Read the model definition and answer for the solid it produces. Units are mm, in the model's axes. Coordinates: 2 decimals unless noted, no trailing zeros. Order: outer loops, then holes, each group sorted by start corner. A loop starts at its lowest first (then second) coordinate and runs counter-clockwise, first axis right, second up. Notation, with made-up numbers: (43.5, 68.5) -> (101.5, 68.5) arc R13 ccw to (101.5, 74.5) -> close; hole circle Ø4 at (74, -31.5). An arc over 180 degrees is marked (long way). Answer as a JSON object with one key per item and string values. Group by question number.
1) Determine the mould class of faces 1 (the cylindrical face through (39.1, 0.86, 0.99)), 2 (the cylindrical face through (0.86, 0.9, 0.99)), 3 (the cylindrical face through (27.776, 30.775, 1.479)), 4 (the cylindrical face through (19.762, 39.715, 2.699)) for opening direction X: released by +X, released by -X, zero draft, split by the parting line, or undercut.
2) Section D-D on y = 36 is taken. Determine the outline of the cut face in (x, z).
3) Section B-B on x = 29 is taken. Determine the outline of the cut face in (y, z), and give its area (3 significant figures).
4) Consider L1, parallel to Y at x = 15.5, z = 2.3; L2, parallel to Y at x = 26, z = 0.85; L3, parallel to X at y = 24.5, z = 1.65. Determine where each line is inside the solid, lowest interval first.
5) Section C-C on x = 36 is taken. Determine the outline of the cut face in (y, z).
6) Section A-A on y = 30 is taken. Determine the outline of the cut face in (x, z), and give its area (3 significant figures).
7) Given pin 1 (19 mm diameter, centred on x = 22, y = 23.5, fed in from +Z); pin 2 (4.5 mm diameter, centred on x = 4, y = 36, fed in from +Z); pin 3 (4 mm diameter, centred on x = 24.5, y = 25, fed in from +Z), each flat-ended and moving along its own axis, determine where each tip first touches the part or whether it passes through.
from build123d import *

# Parameters (mm, degrees)
F0_R     = 1.75
F1_DEPTH = 3
F2_R     = 1


with BuildPart() as f1:
    # F0 (on Top) → F1 (new body)
    with BuildSketch(Plane.XY):
        with BuildLine():
            ThreePointArc((0, 3), (0.8786796564, 0.8786796564), (3, 0))
            Line((3, 0), (37, 0))
            ThreePointArc((37, 0), (39.1213203436, 0.8786796564), (40, 3))
            Line((40, 3), (40, 37))
            ThreePointArc((40, 37), (39.1213203436, 39.1213203436), (37, 40))
            Line((37, 40), (3, 40))
            ThreePointArc((3, 40), (0.8786796564, 39.1213203436), (0, 37))
            Line((0, 37), (0, 3))
        make_face()
        with Locations((4, 4)):
            Circle(F0_R, mode=Mode.SUBTRACT)
        with BuildLine():
            ThreePointArc((25.7168143959, 2.4054544485), (16.6516253204, 1.8055396616), (8.3939355728, 5.5934296756))
            ThreePointArc((8.3939355728, 5.5934296756), (20.1917154021, 6.7967188392), (27.1456707418, 16.4028636876))
            ThreePointArc((27.1456707418, 16.4028636876), (27.9768447331, 19.3917664063), (27.6084521304, 22.472135955))
            ThreePointArc((27.6084521304, 22.472135955), (31.4294663136, 11.9894373312), (25.7168143959, 2.4054544485))
        make_face(mode=Mode.SUBTRACT)
        with BuildLine():
            ThreePointArc((5.0331856041, 9.1259728326), (1.6613352552, 17.56209611), (2.7120662697, 26.5861481412))
            ThreePointArc((2.7120662697, 26.5861481412), (7.5021767329, 15.7376295574), (18.7870537655, 12.0924870261))
            ThreePointArc((18.7870537655, 12.0924870261), (21.8865160613, 12.2256153201), (24.7022820183, 13.527864045))
            ThreePointArc((24.7022820183, 13.527864045), (15.9134015021, 6.6545315855), (5.0331856041, 9.1259728326))
        make_face(mode=Mode.SUBTRACT)
        with Locations((36, 4)):
            Circle(F0_R, mode=Mode.SUBTRACT)
        with BuildLine():
            ThreePointArc((20, 28), (31.1503971529, 28.3946684161), (38.5, 20))
            ThreePointArc((38.5, 20), (36.2692553858, 11.1931089939), (30.1149914386, 4.5101017371))
            ThreePointArc((30.1149914386, 4.5101017371), (32.6163099018, 16.1022939223), (25.6292136254, 25.6843604706))
            ThreePointArc((25.6292136254, 25.6843604706), (23.0434451067, 27.3984756459), (20, 28))
        make_face(mode=Mode.SUBTRACT)
        with BuildLine():
            ThreePointArc((5.0331856041, 30.8740271674), (12.014456559, 36.687752873), (20.9215337867, 38.4770337306))
            ThreePointArc((20.9215337867, 38.4770337306), (12.0842050334, 30.5689913546), (12.1046872588, 18.7100245281))
            ThreePointArc((12.1046872588, 18.7100245281), (13.1890863131, 15.8033996199), (15.2977179817, 13.527864045))
            ThreePointArc((15.2977179817, 13.527864045), (6.0448769164, 19.7626095929), (5.0331856041, 30.8740271674))
        make_face(mode=Mode.SUBTRACT)
        with Locations((4, 36)):
            Circle(F0_R, mode=Mode.SUBTRACT)
        with BuildLine():
            ThreePointArc((25.7168143959, 37.5945455515), (33.4033274796, 32.7515023614), (37.8574729322, 24.8332867156))
            ThreePointArc((37.8574729322, 24.8332867156), (27.6055929298, 30.7943663266), (16.3333746086, 27.1102642876))
            ThreePointArc((16.3333746086, 27.1102642876), (13.9041077858, 25.1807430078), (12.3915478696, 22.472135955))
            ThreePointArc((12.3915478696, 22.472135955), (15.461858115, 33.1987530743), (25.7168143959, 37.5945455515))
        make_face(mode=Mode.SUBTRACT)
        with Locations((36, 36)):
            Circle(F0_R, mode=Mode.SUBTRACT)
    extrude(amount=F1_DEPTH)

    # F2
    f2_edges = [f1.edges().sort_by_distance(p)[0] for p in [
        (20, 0, 3),
    ]]
    fillet(f2_edges, radius=F2_R)

    # F4 (on offset) → F5 (revolve)
    with BuildSketch(Plane.XZ.offset(-20)):
        with BuildLine():
            Line((12, 3), (20, 3))
            Line((20, 3), (20, 4.5))
            ThreePointArc((20, 4.5), (16.1031638738, 4.2209285699), (12.292759493, 3.358356189))
            ThreePointArc((12.292759493, 3.358356189), (12.1024290926, 3.2150836308), (12, 3))
        make_face()
    revolve(axis=Axis((20, 20, 2.25), (0, 0, 1)))


solid = f1.part
Worked answers:
{
 "1": {"face 1": "released by +X", "face 2": "released by -X", "face 3": "undercut", "face 4": "zero draft"},
 "2": {"outline": "(0, 0) -> (2.25, 0) -> (2.25, 3) -> (1, 3) arc R1 ccw to (0, 2) -> close; (5.75, 0) -> (10.71, 0) -> (10.71, 3) -> (5.75, 3) -> close; (16.29, 0) -> (18.96, 0) -> (18.96, 3) -> (16.29, 3) -> close; (29.29, 0) -> (34.25, 0) -> (34.25, 3) -> (29.29, 3) -> close; (37.75, 0) -> (40, 0) -> (40, 2) arc R1 ccw to (39, 3) -> (37.75, 3) -> close"},
 "3": {"outline": "(0, 0) -> (5.56, 0) -> (5.56, 3) -> (1, 3) arc R1 ccw to (0, 2) -> close; (20.86, 0) -> (23.02, 0) -> (23.02, 3) -> (20.86, 3) -> close; (29.11, 0) -> (30.58, 0) -> (30.58, 3) -> (29.11, 3) -> close; (36.16, 0) -> (40, 0) -> (40, 2) arc R1 ccw to (39, 3) -> (36.16, 3) -> close", "area": "38.7 mm²"},
 "4": {"L1": "y = 0.05 to 2.06, 5.08 to 6.57, 12.11 to 26.61, 33.24 to 35.32, 37.94 to 39.95", "L2": "y = 0 to 2.6, 13.04 to 25.46, 29.46 to 30.87, 37.5 to 40", "L3": "x = 0 to 2.06, 2.85 to 4.37, 10.83 to 12.22, 13.39 to 27.39, 36.21 to 40"},
 "5": {"outline": "(0, 0) -> (2.25, 0) -> (2.25, 3) -> (1, 3) arc R1 ccw to (0, 2) -> close; (5.75, 0) -> (10.71, 0) -> (10.71, 3) -> (5.75, 3) -> close; (24.76, 0) -> (26.95, 0) -> (26.95, 3) -> (24.76, 3) -> close; (29.29, 0) -> (34.25, 0) -> (34.25, 3) -> (29.29, 3) -> close; (37.75, 0) -> (40, 0) -> (40, 2) arc R1 ccw to (39, 3) -> (37.75, 3) -> close"},
 "6": {"outline": "(0, 0) -> (4.75, 0) -> (4.75, 3) -> (1, 3) arc R1 ccw to (0, 2) -> close; (11.84, 0) -> (13.39, 0) -> (13.39, 3) -> (11.84, 3) -> close; (21.12, 0) -> (31.04, 0) -> (31.04, 3) -> (21.12, 3) -> close; (35.56, 0) -> (40, 0) -> (40, 2) arc R1 ccw to (39, 3) -> (35.56, 3) -> close", "area": "61.5 mm²"},
 "7": {"pin 1": "stops at z = 4.5", "pin 2": "stops at z = 3", "pin 3": "stops at z = 4.08"}
}
